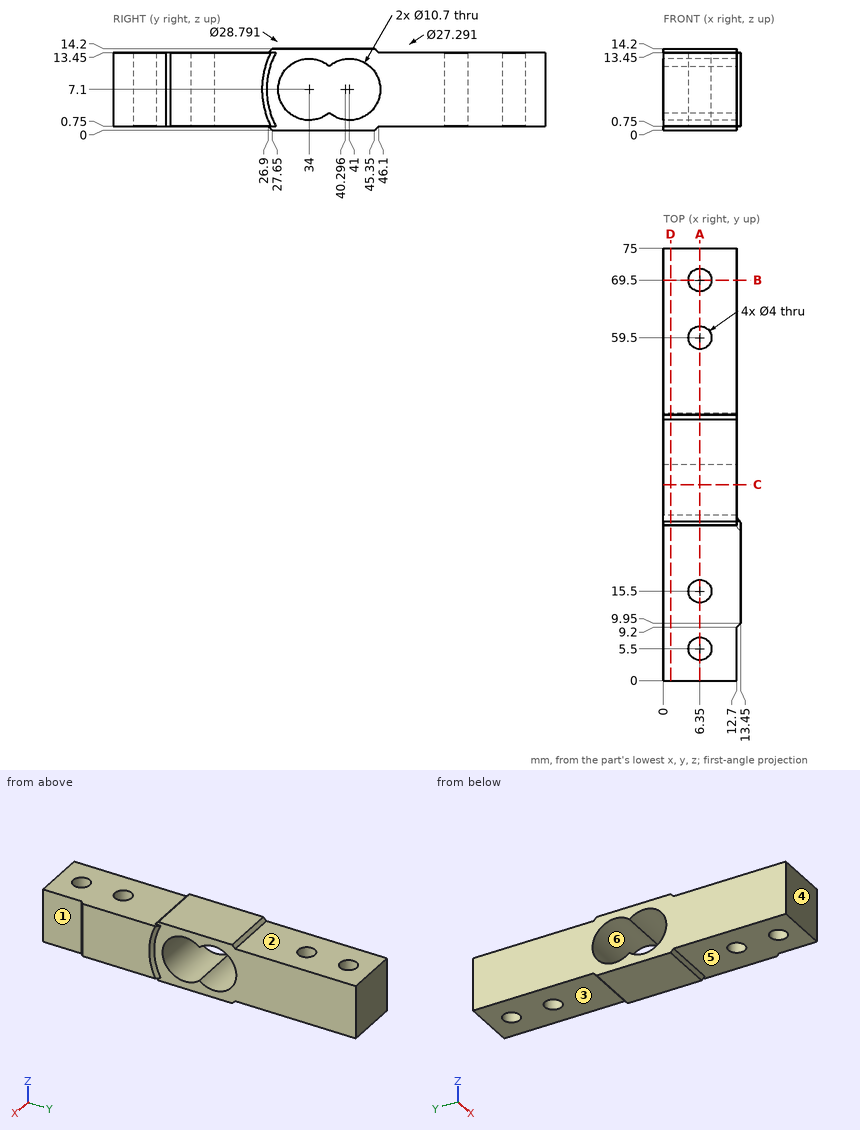
Could you check a few things on this drawing? It's one solid part, dimensions in mm from its lowest x, y, z. A direction names the side the tool comes from. Give positions to 0.01 mm unless a question says otherwise; leave off trailing zeros. Loops run counter-clockwise (first coordinate to the right, second up) from the corner with the lowest first, then second, coordinate; pieces in that order, holes last. Notation, with made-up numbers: (17.5, 11.5) -> (51.5, 11.5) arc R30 ccw to (51.5, 49.5) -> close; hole circle Ø3 at (19.5, 36). An arc over 180 degrees is marked (long way). Answer as CSV lines item,"result". Start each with the question number.
(1) I need wall thicknesses on probe 1 along Z at (x, y) = (9.5, 34); probe 2 along X at (y, z) = (15.5, 6.75); probe 3 along X at (y, z) = (5.5, 3.5). Which ranges of each line are inside material? Lowest first, please.
(2) We'd pull the mould along Y, two halves only. Please class the marked faces 4, 5 and 6: released by +Y, released by -Y, zero draft, split by the parting line, or undercut.
(3) If we section it at D-D on x = 1.25: Write out the boundary of the cut face in (y, z).
(4) If we section it at A-A on x = 6.35: Count the separate pieces of the cut face and the enclosed holes in it, then the cut area to 3 significant figures.
(5) Which directions (+Z, -Z, +X, -X, +Y, -Y) give clear straight access to the entire face, cutting with the end or side of a thin tool? Please do the marked faces 1, 2 and 3.
(6) If we section it at C-C on y = 34: Write out the boundary of the cut face in (x, z).
(7) I'm going to push flat-ended pins straight in: pin 1 Ø8 at (x, y) = (5, 8.5) entering from +Z; pin 2 Ø4 at (x, y) = (3.5, 63.5) entering from -Z; pin 3 Ø4.5 at (y, z) = (6.5, 4.5) entering from +X. Where does each tip first touch, or does it pass through?
(8) If we section it at B-B on y = 69.5: Write out the boundary of the cut face in (x, z).
Computed:
1,probe 1,"z = 0 to 1.75, 12.45 to 14.2"
1,probe 2,"x = 0 to 4.35, 8.35 to 13.45"
1,probe 3,"x = 0 to 4.35, 8.35 to 12.7"
2,face 4,"released by -Y"
2,face 5,"zero draft"
2,face 6,"undercut"
3,outline,"(0, 0.75) -> (26.9, 0.75) -> (27.65, 0) -> (45.35, 0) -> (46.1, 0.75) -> (75, 0.75) -> (75, 13.45) -> (46.1, 13.45) -> (45.35, 14.2) -> (27.65, 14.2) -> (26.9, 13.45) -> (0, 13.45) -> close; hole (37.5, 3.05) arc R5.35 ccw (long way) to (37.5, 11.15) arc R5.35 ccw (long way) to start"
4,separate pieces,"5"
4,enclosed holes,"1"
4,area,"618 mm2"
5,face 1,"+Z, -Z, +X, -Y"
5,face 2,"+Z, +X, -X, +Y"
5,face 3,"-Z, +X, -X, +Y"
6,outline,"(0, 0) -> (12.7, 0) -> (12.7, 1.75) -> (0, 1.75) -> close; (0, 12.45) -> (12.7, 12.45) -> (12.7, 14.2) -> (0, 14.2) -> close"
7,pin 1,"stops at z = 13.45"
7,pin 2,"stops at z = 0.75"
7,pin 3,"stops at x = 12.7"
8,outline,"(0, 0.75) -> (4.35, 0.75) -> (4.35, 13.45) -> (0, 13.45) -> close; (8.35, 0.75) -> (12.7, 0.75) -> (12.7, 13.45) -> (8.35, 13.45) -> close"
